Geometry: final body of the model. Coordinates: model frame, mm. Face numbers are marked on the shaded views. A direction names the side the tool comes from. Give positions to 0.01 mm unless a question says otherwise; leave off trailing zeros. Loops run counter-clockwise (first coordinate to the right, second up) from the corner with the lowest first, then second, coordinate; pieces in that order, holes last. Notation, with made-up numbers: (-3.5, -36.75) - (42.5, -36.75) arc R12 ccw to (42.5, -29.75) - close; hole circle Ø6 at (-7, 30.5). An arc over 180 degrees is marked (long way). Answer in a Markdown table with one row per item.
from build123d import *

# Parameters (mm, degrees)
F1_DEPTH = 20


with BuildPart() as f1:
    # F0 (on Top) → F1 (new body)
    with BuildSketch(Plane.XY):
        with BuildLine():
            Line((-41.75, -120.5), (0, -120.5))
            Line((0, -120.5), (41.75, -120.5))
            ThreePointArc((41.75, -120.5), (43.164214, -119.914214), (43.75, -118.5))
            Line((43.75, -118.5), (43.75, -106.5))
            Line((43.75, -106.5), (55, -106.5))
            ThreePointArc((55, -106.5), (58.535534, -105.035534), (60, -101.5))
            Line((60, -101.5), (60, 48.5))
            ThreePointArc((60, 48.5), (58.535534, 52.035534), (55, 53.5))
            Line((55, 53.5), (43.75, 53.5))
            Line((43.75, 53.5), (43.75, 76.75))
            ThreePointArc((43.75, 76.75), (30.935922, 107.685922), (0, 120.5))
            ThreePointArc((0, 120.5), (-30.935922, 107.685922), (-43.75, 76.75))
            Line((-43.75, 76.75), (-43.75, 53.5))
            Line((-43.75, 53.5), (-55, 53.5))
            ThreePointArc((-55, 53.5), (-58.535534, 52.035534), (-60, 48.5))
            Line((-60, 48.5), (-60, -101.5))
            ThreePointArc((-60, -101.5), (-58.535534, -105.035534), (-55, -106.5))
            Line((-55, -106.5), (-43.75, -106.5))
            Line((-43.75, -106.5), (-43.75, -118.5))
            ThreePointArc((-43.75, -118.5), (-43.164214, -119.914214), (-41.75, -120.5))
        make_face()
        with BuildLine():
            Line((-45.750001, -120.5), (-41.75, -120.5))
            ThreePointArc((-41.75, -120.5), (-43.164214, -119.914214), (-43.75, -118.5))
            Line((-43.75, -118.5), (-43.75, -106.5))
            Line((-43.75, -106.5), (-55, -106.5))
            ThreePointArc((-55, -106.5), (-58.535534, -105.035534), (-60, -101.5))
            Line((-60, -101.5), (-60, 48.5))
            ThreePointArc((-60, 48.5), (-58.535534, 52.035534), (-55, 53.5))
            Line((-55, 53.5), (-43.75, 53.5))
            Line((-43.75, 53.5), (-43.75, 76.75))
            ThreePointArc((-43.75, 76.75), (-30.935922, 107.685922), (0, 120.5))
            ThreePointArc((0, 120.5), (30.935922, 107.685922), (43.75, 76.75))
            Line((43.75, 76.75), (43.75, 53.5))
            Line((43.75, 53.5), (55, 53.5))
            ThreePointArc((55, 53.5), (58.535534, 52.035534), (60, 48.5))
            Line((60, 48.5), (60, -101.5))
            ThreePointArc((60, -101.5), (58.535534, -105.035534), (55, -106.5))
            Line((55, -106.5), (43.75, -106.5))
            Line((43.75, -106.5), (43.75, -118.5))
            ThreePointArc((43.75, -118.5), (43.164214, -119.914214), (41.75, -120.5))
            Line((41.75, -120.5), (45.750001, -120.5))
            ThreePointArc((45.750001, -120.5), (47.871322, -119.62132), (48.750001, -117.5))
            Line((48.750001, -117.5), (48.750001, -111.500001))
            Line((48.750001, -111.500001), (55, -111.500001))
            ThreePointArc((55, -111.500001), (62.071069, -108.571069), (65.000001, -101.5))
            Line((65.000001, -101.5), (65.000001, 48.5))
            ThreePointArc((65.000001, 48.5), (62.071069, 55.571069), (55, 58.500001))
            Line((55, 58.500001), (48.750001, 58.500001))
            Line((48.750001, 58.500001), (48.750001, 76.75))
            ThreePointArc((48.750001, 76.75), (34.471456, 111.221456), (0, 125.500001))
            ThreePointArc((0, 125.500001), (-34.471456, 111.221456), (-48.750001, 76.75))
            Line((-48.750001, 76.75), (-48.750001, 58.500001))
            Line((-48.750001, 58.500001), (-55, 58.500001))
            ThreePointArc((-55, 58.500001), (-62.071069, 55.571069), (-65.000001, 48.5))
            Line((-65.000001, 48.5), (-65.000001, -101.5))
            ThreePointArc((-65.000001, -101.5), (-62.071069, -108.571069), (-55, -111.500001))
            Line((-55, -111.500001), (-48.750001, -111.500001))
            Line((-48.750001, -111.500001), (-48.750001, -117.5))
            ThreePointArc((-48.750001, -117.5), (-47.871322, -119.62132), (-45.750001, -120.5))
        make_face()
    extrude(amount=F1_DEPTH)


solid = f1.part
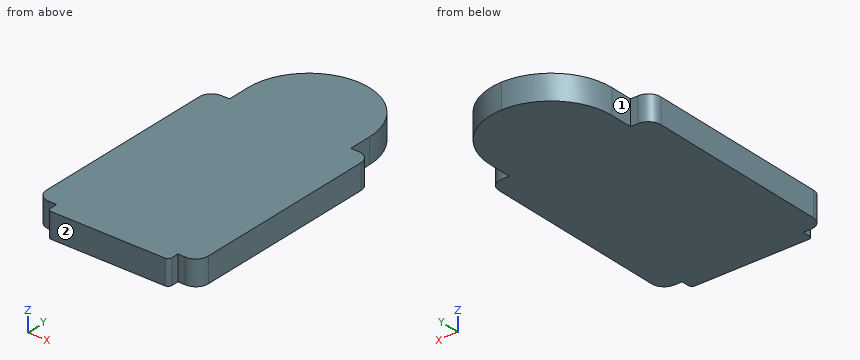
Q1. Cut plane C-C (y = 85). Output: boundary loops of the cut face in (x, z), and give its area (3 significant figures).
Check values:
| item | result |
|---|---|
| outline | (-48.05, 0) - (48.05, 0) - (48.05, 20) - (-48.05, 20) - close |
| area | 1,920 mm² |
Q2. Reachability of the marked faces 1 and 2 from +Z, -Z, +X, -X, +Y, -Y: full face, straight path, thin tool, end or side. Return the list, or none.
Check values:
| item | result |
|---|---|
| face 1 | +Z, -Z, -X, +Y |
| face 2 | +Z, -Z, +X, -X, -Y |
Q3. Cut plane A-A (z = 8.25). Output: boundary loops of the cut face in (x, y).
Check values:
| item | result |
|---|---|
| outline | (-65, -101.5) arc R10 ccw to (-55, -111.5) - (-48.75, -111.5) - (-48.75, -117.5) arc R3 ccw to (-45.75, -120.5) - (45.75, -120.5) arc R3 ccw to (48.75, -117.5) - (48.75, -111.5) - (55, -111.5) arc R10 ccw to (65, -101.5) - (65, 48.5) arc R10 ccw to (55, 58.5) - (48.75, 58.5) - (48.75, 76.75) arc R48.75 ccw to (0, 125.5) arc R48.75 ccw to (-48.75, 76.75) - (-48.75, 58.5) - (-55, 58.5) arc R10 ccw to (-65, 48.5) - close |
Q4. Cut plane B-B (x = -27.5). Output: boundary loops of the cut face in (y, z).
Check values:
| item | result |
|---|---|
| outline | (-120.5, 0) - (117, 0) - (117, 20) - (-120.5, 20) - close |
Q5. First-contact query: pin 1 (2 mm diameter, centred on x = -25.5, y = 81.5, fed in from -Z); pin 2 (1.8 mm diameter, centred on y = -114.5, z = 6, fed in from +X); pin 3 (5 mm diameter, centred on x = 50.5, z = 8.5, fed in from -Y); pin 4 (2 mm diameter, centred on x = -43.5, z = 12, fed in from +Y). Flat tips, straight axial feed; report the tip coordinate or a pass-through.
Check values:
| item | result |
|---|---|
| pin 1 | z = 0 |
| pin 2 | x = 48.75 |
| pin 3 | y = -119.48 |
| pin 4 | y = 100.63 |
Q6. Material intervals for line 1 along Y through (x, z) = (-56, 1.75); line 2 along X through (y, z) = (70.5, 2); line 3 along Y through (x, z) = (50.5, 17.5), sorted ascending.
Check values:
| item | result |
|---|---|
| line 1 | -111.45 to 58.45 |
| line 2 | -48.75 to 48.75 |
| line 3 | -111.5 to 58.5 |
